from build123d import *

# Parameters (mm, degrees)
F0_R     = 28.575
F2_DEPTH = 3.175
F1_R     = 22.6695
F3_DEPTH = 6.35
F4_R     = 1.4432349382
F5_DEPTH = 6.351


# Not quite as in the source:
# - a fillet or chamfer that OpenCascade refuses, or shapes differently, is made with other operations: its cross-section is extruded or revolved along the edge and cut away or added


with BuildPart() as f2:
    # F0 (on Top) → F2 (new body)
    with BuildSketch(Plane.XY):
        Circle(F0_R)
    extrude(amount=F2_DEPTH)

    # F1 (on Top) → F3 (join)
    with BuildSketch(Plane.XY):
        Circle(F1_R)
    extrude(amount=F3_DEPTH)

    # F4 (on face) → F5 (cut, through all)
    with BuildSketch(Plane.XY.offset(6.35)):
        with Locations((0, 25.9878132492)):
            Circle(F4_R)
    extrude(amount=-F5_DEPTH, mode=Mode.SUBTRACT)

    # F6: fillet of radius 12.7 on 1 edges, made by hand

    # F6_s1 → F6_t2 (revolve, cut)
    with BuildSketch(Plane.XZ):
        with BuildLine():
            ThreePointArc((22.6695, 3.175), (18.7593676479, 5.529762203), (14.2692395874, 6.35))
            Line((14.2692395874, 6.35), (14.2692395874, 6.604))
            Line((14.2692395874, 6.604), (22.6695, 6.604))
            Line((22.6695, 6.604), (22.9235, 6.35))
            ThreePointArc((22.9235, 6.35), (22.9235, 4.7625), (22.8375052083, 3.3655))
            Line((22.8375052083, 3.3655), (22.6695, 3.175))
        make_face()
    revolve(axis=Axis((0, 0, 6.35), (0, 0, 1)), mode=Mode.SUBTRACT)


solid = f2.part
Geometry: final body of the model. Coordinates: model frame, mm. A direction names the side the tool comes from. Round coordinates to 2 decimals unless told otherwise and drop trailing zeros. Loops run counter-clockwise (first coordinate to the right, second up) from the corner with the lowest first, then second, coordinate; pieces in that order, holes last. Notation, with made-up numbers: (-36.75, 88.25) - (-28.75, 88.25) arc R24 ccw to (-28.75, 123.25) - close; hole circle Ø6 at (43.25, 24). An arc over 180 degrees is marked (long way). Write each question's results on one line, items separated by ' | '. Start each with the question number.
1) First-contact query: P1, Ø3, axis at x = 10.5, z = 5.5, coming from the +Y side; P2, Ø6, axis at x = -12, y = 18.5, coming from the +Z side; P3, Ø2, axis at x = -8, z = 5.5, coming from the -Y side. Flat tips, straight axial feed; report the tip coordinate or a pass-through.
2) Access query for faces 4 (the face through (-9, 21, 3.175)), 5 (the face through (0, 0, 6.35)). Directions: +Z, -Z, +X, -X, +Y, -Y. A direction counts if a zero-diameter tool reaches every point of the face in a straight line with its end or side. Return the directions, or none.
3) Mould query, pull axis X, two halves, no side actions, for faces 1 (the face through (-0.19, 27.42, 1.61)), 2 (the face through (-28.547, 1.256, 1.565)), 3 (the face through (0, 0, 0)). Classes: released by +X, released by -X, zero draft, split by the parting line, or undercut.
4) Line query: probe 1 along Y at (x, z) = (0, 1.05) (3 decimals); probe 2 along Z at (x, y) = (-13.5, 23.5) (3 decimals); probe 3 along Z at (x, y) = (4.5, -15.5). Output: solid intervals per line, ascending. Write a range as [from, to].
5) Cut plane C-C on z = 5.5. Return loops of the section in (x, y).
Verdict:
1) P1: stops at y = 19.04 | P2: stops at z = 5.42 | P3: stops at y = -19.32
2) face 4: +Z | face 5: +Z, +X, -X, +Y, -Y
3) face 1: undercut | face 2: split by the parting line | face 3: zero draft
4) probe 1: y = [-28.575, 24.545], [27.431, 28.575] | probe 2: z = [0, 3.175] | probe 3: z = [0, 6.21]
5) outline: circle Ø37.67 at (0, 0)
